Read the model definition and answer for the solid it produces. Units are mm, in the model's axes. A direction names the side the tool comes from. Give positions to 0.01 mm unless a question says otherwise; leave off trailing zeros. Write each loop counter-clockwise with the first axis right and the second up, starting at its lowest first coordinate (ties: lowest second). Pieces come first, ordered by that corner, then holes. Notation, with made-up numbers: M -22,-33 L 11,-33 A17 cw 11,-17 Z; hole C 76,29.25 d5. An arc over 180 degrees is marked long. Use a Markdown table: item, result. Add a question column.
Item 1: A cutting plane is placed at B-B on y = 2. Count the separate pieces of the cut face and the enclosed holes in it, then the cut area to 3 significant figures.
Item 2: A cutting plane is placed at D-D on z = -93.5. Determine the outline of the cut face in (x, y).
Item 3: For faces 4 (the flat face through (20, 12.7, 20)), 5 (the flat face through (111, 10.033, -46)), determine the directions among +Z, -Z, +X, -X, +Y, -Y from which every point of the face is accessible in a straight line to the end or side of a thin tool.
Item 4: The mould has two halves that part along Z. Classify faces 1 (the cylindrical face through (48.13, 6.26, 116.84)), 2 (the flat face through (111, 10.033, 46)), 3 (the cylindrical face through (-116.652, 6.261, -48.584)): pulls with the +Z half, pulls with the -Z half, needs draft (parallel to the pull), parting line crosses it, or undercut.
Item 5: A cutting plane is placed at A-A on z = 16.5. Determine the outline of the cut face in (x, y), then the cut area to 3 significant figures.
Item 6: A cutting plane is placed at C-C on x = -89. Determine the outline of the cut face in (y, z).
Item 7: Consider probe 1 along X at (y, z) = (10.7, 0); probe 2 along X at (y, z) = (10, -34.5); probe 3 along Z at (x, y) = (12, 11.25). Determine where each line is inside the solid, lowest interval first. Write a range as [from, to].
Item 8: Given P1, Ø1, axis at y = 11.5, z = -81, coming from the -X side; P2, Ø4, axis at x = -47.07, z = -113.64, coming from the +Y side; P3, Ø7.5, axis at x = -47, z = 114, coming from the +Y side; P4, Ø4, axis at x = -51.27, z = -51.27, coming from the +Y side, each flat-ended and moving along its own axis, determine where each tip first touches the part or whether it passes through.
from build123d import *

# Parameters (mm, degrees)
BOSS_EXTRUDE1_DEPTH                                 = 12.7
SKETCH3_R                                           = 24.5745
CUT_EXTRUDE1_DEPTH                                  = 174.423960282
SKETCH5_R                                           = 51.3715
SKETCH5_R_2                                         = 46.5455
CUT_EXTRUDE2_DEPTH                                  = 2.794
CIRPATTERN4_COUNT                                   = 8
CBORE_FOR_8_BINDING_HEAD_MACHINE_SCREW2_D           = 4.4958
CBORE_FOR_8_BINDING_HEAD_MACHINE_SCREW2_CBORE_D     = 9.525
CBORE_FOR_8_BINDING_HEAD_MACHINE_SCREW2_CBORE_DEPTH = 2.667
CIRPATTERN5_COUNT                                   = 8


with BuildPart() as part:
    # Sketch1 → Boss-Extrude1 (new body)
    with BuildSketch(Plane(origin=(0, 0, 0), x_dir=(1, 0, 0), z_dir=(0, 1, 0))):
        with BuildLine():
            ThreePointArc((-31.793446259, 122.3), (-48.357791931, 116.746037126), (-63.997797892, 108.960520786))
            Line((-63.997797892, 108.960520786), (-108.960520786, 63.997797892))
            ThreePointArc((-108.960520786, 63.997797892), (-116.746037126, 48.357791931), (-122.3, 31.793446259))
            Line((-122.3, 31.793446259), (-122.3, -31.793446259))
            ThreePointArc((-122.3, -31.793446259), (-116.746037126, -48.357791931), (-108.960520786, -63.997797892))
            Line((-108.960520786, -63.997797892), (-63.997797892, -108.960520786))
            ThreePointArc((-63.997797892, -108.960520786), (-48.357791931, -116.746037126), (-31.793446259, -122.3))
            Line((-31.793446259, -122.3), (31.793446259, -122.3))
            ThreePointArc((31.793446259, -122.3), (48.357791931, -116.746037126), (63.997797892, -108.960520786))
            Line((63.997797892, -108.960520786), (108.960520786, -63.997797892))
            ThreePointArc((108.960520786, -63.997797892), (116.746037126, -48.357791931), (122.3, -31.793446259))
            Line((122.3, -31.793446259), (122.3, 31.793446259))
            ThreePointArc((122.3, 31.793446259), (116.746037126, 48.357791931), (108.960520786, 63.997797892))
            Line((108.960520786, 63.997797892), (63.997797892, 108.960520786))
            ThreePointArc((63.997797892, 108.960520786), (48.357791931, 116.746037126), (31.793446259, 122.3))
            Line((31.793446259, 122.3), (-31.793446259, 122.3))
        make_face()
    extrude(amount=BOSS_EXTRUDE1_DEPTH)

    # Sketch3 → Cut-Extrude1 (cut, through all)
    with BuildSketch(Plane(origin=(0, 12.7, 0), x_dir=(1, 0, 0), z_dir=(0, 1, 0))):
        with Locations(Location((0, 0, 0), (0, 0, 270))):
            Circle(SKETCH3_R)
    extrude(amount=-CUT_EXTRUDE1_DEPTH, mode=Mode.SUBTRACT)

    # Sketch5 → Cut-Extrude2 (cut)
    with BuildSketch(Plane(origin=(0, 12.7, 0), x_dir=(1, 0, 0), z_dir=(0, 1, 0))):
        with Locations(Location((0, 0, 0), (0, 0, 270))):
            Circle(SKETCH5_R)
        with Locations(Location((0, 0, 0), (0, 0, 270))):
            Circle(SKETCH5_R_2, mode=Mode.SUBTRACT)
    extrude(amount=-CUT_EXTRUDE2_DEPTH, mode=Mode.SUBTRACT)

    # Sketch23 → M8x1.25 Tapped Hole1 (revolve, cut)
    with BuildSketch(Plane(origin=(-72.5, 12.7, 0), x_dir=(0, 0, 1), z_dir=(1, 0, 0))):
        Polygon((0, 0), (0, 8.392926105), (3.4, 6.35), (3.4, 0), align=None)
    m8x1_25_tapped_hole1 = revolve(axis=Axis((-72.5, 19.05, 0), (0, -1, 0)), mode=Mode.SUBTRACT)

    # CirPattern4: M8x1.25 Tapped Hole1 ×8 about axis
    cirpattern4_axis = Axis((0, 0, 0), (0, 1, 0))
    for i in range(1, CIRPATTERN4_COUNT):
        add(m8x1_25_tapped_hole1.rotate(cirpattern4_axis, i * 360 / CIRPATTERN4_COUNT), mode=Mode.SUBTRACT)

    # CBORE for #8 Binding Head Machine Screw2 (through all)
    with Locations(Plane(origin=(0, 12.7, 0), x_dir=(1, 0, 0), z_dir=(0, 1, 0))):
        with Locations((-47.069870839, 113.636720559)):
            cbore_for_8_binding_head_machine_screw2 = CounterBoreHole(CBORE_FOR_8_BINDING_HEAD_MACHINE_SCREW2_D / 2, CBORE_FOR_8_BINDING_HEAD_MACHINE_SCREW2_CBORE_D / 2, CBORE_FOR_8_BINDING_HEAD_MACHINE_SCREW2_CBORE_DEPTH)

    # CirPattern5: CBORE for #8 Binding Head Machine Screw2 ×8 about axis
    cirpattern5_axis = Axis((0, 0, 0), (0, 1, 0))
    for i in range(1, CIRPATTERN5_COUNT):
        add(cbore_for_8_binding_head_machine_screw2.rotate(cirpattern5_axis, i * 360 / CIRPATTERN5_COUNT), mode=Mode.SUBTRACT)


solid = part.part
Filled in:
| question | item | result |
|---|---|---|
| 1 | separate pieces | 1 |
| 1 | enclosed holes | 9 |
| 1 | area | 46,800 mm² |
| 2 | outline | M -79.46,0 L 79.46,0 L 79.46,12.7 L -79.46,12.7 Z |
| 3 | face 4 | +Z, -Z, +X, -X, +Y |
| 3 | face 5 | +Y |
| 4 | face 1 | pulls with the +Z half |
| 4 | face 2 | undercut |
| 4 | face 3 | pulls with the -Z half |
| 5 | outline | M -122.3,0 L -18.21,0 L -18.21,12.7 L -43.52,12.7 L -43.52,9.91 L -48.65,9.91 L -48.65,12.7 L -122.3,12.7 Z; M 18.21,0 L 122.3,0 L 122.3,12.7 L 48.65,12.7 L 48.65,9.91 L 43.52,9.91 L 43.52,12.7 L 18.21,12.7 Z |
| 5 | area | 2,620 mm² |
| 6 | outline | M 0,-83.96 L 12.7,-83.96 L 12.7,83.96 L 0,83.96 Z |
| 7 | probe 1 | [-122.3, -75.9], [-69.1, -51.37], [-46.55, -24.57], [24.57, 46.55], [51.37, 69.1], [75.9, 122.3] |
| 7 | probe 2 | [-121.56, -38.06], [-31.24, 31.24], [38.06, 121.56] |
| 7 | probe 3 | [-122.3, -49.95], [-44.97, -21.45], [21.45, 44.97], [49.95, 122.3] |
| 8 | P1 | x = -92.46 |
| 8 | P2 | through |
| 8 | P3 | y = 10.03 |
| 8 | P4 | y = 5.51 |
